Read the model definition and answer for the solid it produces. Units are mm, in the model's axes. A direction names the side the tool comes from. Round coordinates to 2 decimals unless told otherwise and drop trailing zeros. Order: outer loops, then holes, each group sorted by start corner. A loop starts at its lowest first (then second) coordinate and runs counter-clockwise, first axis right, second up.
Autodesk Inventor part; units mm, degrees
ref_plane "Start plane" through (0, 0, 0) normal (0, 0, 1) x (1, 0, 0)
ref_plane "End plane" through (0, 0, 140) normal (0, 0, 1) x (1, 0, 0)
ref_plane "YZ Plane" through (0, 0, 0) normal (1, 0, 0) x (0, 1, 0)
ref_plane "Start plane" through (0, 0, 0) normal (0, 0, 1) x (1, 0, 0)
ref_plane "End plane" through (0, 0, 140) normal (0, 0, 1) x (1, 0, 0)
sketch "Sketch" plane through (0, 0, 0) normal (0, 0, 1) x (1, 0, 0)
  line L0 (-1.6, 0) -> (-1.6, 60)
  line L1 (-1.6, 60) -> (53.4, 60)
  line L2 (53.4, 60) -> (53.4, 58.1111)
  line L3 (49.3704, 53.6358) -> (11.8638, 49.6937)
  line L4 (4.7, 41.7375) -> (4.7, 0)
  line L5 (4.7, 0) -> (-1.6, 0) construction
  line L6 (29.05, 60) -> (29.05, 51.5) construction
  line L7 (53.4, 54.0593) -> (53.4, 51.5) construction
  line L8 (53.4, 51.5) -> (29.05, 51.5) construction
  line L9 (0, 15) -> (0, -27) construction
  line L10 (-5.539, 0) -> (16.0067, 0) construction
  line L11 (-1.6, 0) -> (-1.6, -60)
  line L12 (-1.6, -60) -> (53.4, -60)
  line L13 (53.4, -60) -> (53.4, -58.1111)
  line L14 (49.3704, -53.6358) -> (11.8638, -49.6937)
  line L15 (4.7, -41.7375) -> (4.7, 0)
  arc A0 (11.8638, 49.6937) -> (4.7, 41.7375) centre (12.7, 41.7375) ccw
  arc A1 (4.7, -41.7375) -> (11.8638, -49.6937) centre (12.7, -41.7375) ccw
  arc A2 (49.3704, 53.6358) -> (53.4, 58.1111) centre (48.9, 58.1111) ccw
  arc A3 (53.4, -58.1111) -> (49.3704, -53.6358) centre (48.9, -58.1111) ccw
  line L16 (0, 23.4) -> (0, -35.4) construction
  line L17 (-9.8481, 0) -> (20.3158, 0) construction
  point P0 (4.7, 48.9407)
  point P1 (53.4, -54.0593)
  point P2 (4.7, -48.9407)
  point P3 (29.05, -60)
  point P4 (29.05, -51.5)
  dimension "d0" = 6.3
  dimension "d1" = 60
  dimension "d2" = 55
  dimension "d3" = 8.5
  dimension "d4" = 24.35
  dimension "d5" = 2.5593
  dimension "d23" = 8
  dimension "d24" = 4.5
  dimension "d25" = 1.6
extrude "Body" add sketch "Sketch" along normal up to surface (140 mm away) from surface at 0
sketch "Sketch3" plane through (0, 0, 0) normal (0, 0, 1) x (1, 0, 0)
  line L0 (0, 0) -> (10, 0)
ref_plane "Work Plane3" through (0, 0, 0) normal (0, -1, 0) x (1, 0, 0)
sketch "Sketch5" plane through (-1.6, 60, 0) normal (-1, 0, 0) x (0, 0, 1)
  circle A0 centre (120, -25) radius 8.5
  circle A1 centre (120, -95) radius 8.5
  line L0 (140, -120) -> (140, 0)
  line L1 (140, -60) -> (0, -60)
  dimension "d30" = 17
  dimension "d31" = 20
  dimension "d32" = 70
extrude "Extrusion2" cut sketch "Sketch5" against normal through all
sketch "Sketch4" plane through (0, 0, 0) normal (0, -1, 0) x (1, 0, 0)
  line L0 (-2, 0) -> (12, 0)
  line L1 (-2, 140) -> (12, 140)
  dimension "d29" = 140
equation "\"d0\" = G_T"
equation "\"d1\" = 0.5 * G_H"
equation "\"d2\" = G_W"
equation "\"d3\" = G_T1"
equation "\"d4\" = G_C"
equation "\"d23\" = G_IR"
equation "\"d24\" = G_ER"
equation "\"d25\" = ex"
equation "\"d6\" = G_L"
equation "\"G_W\" = 55"
equation "\"G_T\" = 6.3"
equation "\"G_T1\" = 8.5"
equation "\"G_NG\" = 0.105104"
equation "\"G_ER\" = 4.5"
equation "\"G_IR\" = 8"
equation "\"G_C\" = 24.35"
equation "\"G_L\" = d29"
equation "\"ex\" = 1.6"
equation "\"G_OFFSET_START\" = 0"
equation "\"G_OFFSET_END\" = 0"
properties part number "ISO 657/11 - CH 120 x 12 - 140" material "Steel, Mild"
Q1. A cutting plane is placed at C-C, the plane z = 13. Give the vertices of the cut face in (x, y), plus the area to 3 significant figures.
Outcome:
outline: (-1.6, -60) - (53.4, -60) - (53.4, -58.11) arc R4.5 ccw to (49.37, -53.64) - (11.86, -49.69) arc R8 cw to (4.7, -41.74) - (4.7, 41.74) arc R8 cw to (11.86, 49.69) - (49.37, 53.64) arc R4.5 ccw to (53.4, 58.11) - (53.4, 60) - (-1.6, 60) - close
area: 1,600 mm2
Q2. For a pull along Y with two mould halves and no side action, classify faces 1 (the face through (1.6, 31.74, 127.85)), 2 (the face through (3, 5, 140)), 3 (the face through (30.88, 51.692, 69.02)), 4 (the face through (26, 60, 69)) as released by +Y, released by -Y, zero draft, split by the parting line, or undercut.
Outcome:
face 1: undercut
face 2: zero draft
face 3: undercut
face 4: released by +Y
Q3. A cutting plane is placed at A-A, the plane z = 120. Give the vertices of the cut face in (x, y).
Outcome:
outline: (-1.6, -60) - (53.4, -60) - (53.4, -58.11) arc R4.5 ccw to (49.37, -53.64) - (11.86, -49.69) arc R8 cw to (4.9, -43.5) - (-1.6, -43.5) - close; (-1.6, -26.5) - (4.7, -26.5) - (4.7, 26.5) - (-1.6, 26.5) - close; (-1.6, 43.5) - (4.9, 43.5) arc R8 cw to (11.86, 49.69) - (49.37, 53.64) arc R4.5 ccw to (53.4, 58.11) - (53.4, 60) - (-1.6, 60) - close
Q4. For faces 5 (the face through (30.88, -51.692, 69.02)), 6 (the face through (26, -60, 69)), determine the directions among +Z, -Z, +X, -X, +Y, -Y from which every point of the face is accessible in a straight line to the end or side of a thin tool.
Outcome:
face 5: +Z, -Z, +X
face 6: +Z, -Z, +X, -X, -Y
Q5. A cutting plane is placed at B-B, the plane y = 35. Give the vertices of the cut face in (x, z).
Outcome:
outline: (-1.6, 0) - (4.7, 0) - (4.7, 111.5) - (-1.6, 111.5) - close; (-1.6, 128.5) - (4.7, 128.5) - (4.7, 140) - (-1.6, 140) - close
Q6. Straight lines are drawn through the part: probe 1 along Y at (x, z) = (3.5, 120); probe 2 along Z at (x, y) = (1, 35); probe 3 along Y at (x, z) = (12, 45.5). For each, find the intervals that lie inside material, in ascending order.
Outcome:
probe 1: y = -60 to -43.5, -26.5 to 26.5, 43.5 to 60
probe 2: z = 0 to 111.5, 128.5 to 140
probe 3: y = -60 to -49.71, 49.71 to 60
Q7. A cutting plane is placed at D-D, the plane x = 17. Give the vertices of the cut face in (y, z), plus the area to 3 significant figures.
Outcome:
outline: (-60, 0) - (-50.23, 0) - (-50.23, 140) - (-60, 140) - close; (50.23, 0) - (60, 0) - (60, 140) - (50.23, 140) - close
area: 2,730 mm2
